from build123d import *

# Parameters (mm, degrees)
F0_W     = 114.3
F0_H     = 57.15
F1_DEPTH = 58.674
F2_W     = 114.3
F2_H     = 42.926
F3_DEPTH = 31.75
F5_DEPTH = 15.748
F7_R     = 12.7
F8_DEPTH = 25.4
F9_DEPTH = 58.674


with BuildPart() as f1:
    # F0 (on Front) → F1 (new body)
    with BuildSketch(Plane.XZ):
        with Locations((-29.805122, -8.710917)):
            Rectangle(F0_W, F0_H)
    extrude(amount=F1_DEPTH)

    # F2 (on face) → F3 (cut)
    with BuildSketch(Plane.XY.offset(19.864083)):
        with Locations((-29.805122, -37.211)):
            Rectangle(F2_W, F2_H)
    extrude(amount=-F3_DEPTH, mode=Mode.SUBTRACT)

    # F4 (on face) → F5 (cut)
    with BuildSketch(Plane.XZ.offset(15.748)):
        Polygon((27.344878, 0.814083), (27.344878, 19.864083), (8.294878, 19.864083), align=None)
        Polygon((-67.905122, 19.864083), (-86.955122, 19.864083), (-86.955122, 0.814083), align=None)
    extrude(amount=-F5_DEPTH, mode=Mode.SUBTRACT)

    # F7 (on face) → F8 (cut)
    with BuildSketch(Plane.XY.offset(-11.885917)):
        with Locations((-29.805122, -36.576)):
            Circle(F7_R)
    extrude(amount=-F8_DEPTH, mode=Mode.SUBTRACT)

    # F6 (on face) → F9 (cut)
    with BuildSketch(Plane.XZ.offset(58.674)):
        Polygon((-29.805122, -24.585917), (-29.805122, -37.285917), (1.944878, -37.285917), (14.644878, -24.585917), align=None)
        Polygon((-61.555122, -37.285917), (-29.805122, -37.285917), (-29.805122, -24.585917), (-74.255122, -24.585917), align=None)
    extrude(amount=-F9_DEPTH, mode=Mode.SUBTRACT)


solid = f1.part
The listing builds one solid part. Answer for the finished solid, in the listing's coordinates (mm). A direction names the side the tool comes from. Give positions to 0.01 mm unless a question says otherwise; leave off trailing zeros. Loops run counter-clockwise (first coordinate to the right, second up) from the corner with the lowest first, then second, coordinate; pieces in that order, holes last. Notation, with made-up numbers: M 37,-40 L 84,-40 A21 cw 84,-6 Z; hole C 51,63.5 d3. An arc over 180 degrees is marked long. Answer as CSV lines item,"result".
Item 1: Given pin 1 Ø2 at (x, z) = (-17, 0.5) entering from +Y; pin 2 Ø6 at (x, y) = (-10, -34.5) entering from +Z; pin 3 Ø4 at (x, z) = (-7.5, -7.5) entering from -Y; pin 4 Ø1 at (x, y) = (-54, -29.5) entering from -Z, each flat-ended and moving along its own axis, determine where each tip first touches the part or whether it passes through.
Values follow:
pin 1,"stops at y = 0"
pin 2,"stops at z = -11.89"
pin 3,"stops at y = -15.75"
pin 4,"stops at z = -24.59"
Item 2: The mould has two halves that part along Z. Classify faces 1 (the cylindrical face through (-31.458, -23.984, -18.147)), 2 (the flat face through (-74, -29, -37.286)), 3 (the flat face through (-67.99, -29.75, -30.85)): released by +Z, released by -Z, zero draft, split by the parting line, or undercut.
Values follow:
face 1,"zero draft"
face 2,"released by -Z"
face 3,"undercut"
Item 3: The part is cut by section C-C (x = -37.5). Give the vertices of the cut face in (y, z).
Values follow:
outline,"M -58.67,-24.59 L -46.68,-24.59 L -46.68,-11.89 L -58.67,-11.89 Z; M -26.47,-24.59 L 0,-24.59 L 0,19.86 L -15.75,19.86 L -15.75,-11.89 L -26.47,-11.89 Z"
Item 4: Straight lines are drawn through the part: line 1 along Z through (x, y) = (-58, -51); line 2 along Z through (x, y) = (-80.5, -33); line 3 along Y through (x, z) = (-18.5, -19). For each, find the intervals that lie inside material, in ascending order. Write a range as [from, to].
Values follow:
line 1,"z = [-24.59, -11.89]"
line 2,"z = [-37.29, -11.89]"
line 3,"y = [-58.67, -42.36], [-30.79, 0]"
Item 5: Which of the six approach directions +Z, -Z, +X, -X, +Y, -Y give full straight-line access (tool end or side, diameter ignored) to faces 4 (the flat face through (17.69, -7.98, 10.47)), 5 (the flat face through (-31, -15.748, 4)), 6 (the flat face through (8.21, -29.75, -31.02))?
Values follow:
face 4,"+Z, +X, +Y, -Y"
face 5,"+Z, +X, -X, -Y"
face 6,"+Y, -Y"
Item 6: The part is cut by section B-B (z = -32.5). Give the vertices of the cut face in (x, y), and give its area (3 significant figures).
Values follow:
outline,"M -86.96,-58.67 L -66.34,-58.67 L -66.34,0 L -86.96,0 Z; M 6.73,-58.67 L 27.34,-58.67 L 27.34,0 L 6.73,0 Z"
area,"2,420 mm^2"
Item 7: The part is cut by section A-A (y = -46.5). Give the vertices of the cut face in (x, z), and give its area (3 significant figures).
Values follow:
outline,"M -86.96,-37.29 L -61.56,-37.29 L -74.26,-24.59 L -37.73,-24.59 L -37.73,-11.89 L -86.96,-11.89 Z; M -21.88,-24.59 L 14.64,-24.59 L 1.94,-37.29 L 27.34,-37.29 L 27.34,-11.89 L -21.88,-11.89 Z"
area,"1,730 mm^2"
Item 8: The part is cut by section D-D (y = -8.5). Give the vertices of the cut face in (x, z).
Values follow:
outline,"M -86.96,-37.29 L -61.56,-37.29 L -74.26,-24.59 L 14.64,-24.59 L 1.94,-37.29 L 27.34,-37.29 L 27.34,0.81 L 8.29,19.86 L -67.91,19.86 L -86.96,0.81 Z"
